Geometry: final body of the model. Coordinates: model frame, mm. Face numbers are marked on the shaded views. A direction names the side the tool comes from. Give positions to 0.01 mm unless a question says otherwise; leave off trailing zeros. Order: outer loops, then holes, each group sorted by start corner. A loop starts at its lowest first (then second) coordinate and runs counter-clockwise, first axis right, second up. Notation, with made-up numbers: (7.5, -31) -> (45.5, -31) arc R17 cw to (45.5, -26) -> close; hole circle Ø4 at (13.25, -23.75). An arc over 180 degrees is marked (long way). One line per question, with ' | ' between items.
from build123d import *

# Parameters (mm, degrees)
SKETCH1_W           = 60
SKETCH1_H           = 25
BOSS_EXTRUDE1_DEPTH = 6
CUT_EXTRUDE3_DEPTH  = 3
SKETCH5_R           = 1.15
CUT_EXTRUDE4_DEPTH  = 33.638167841
SKETCH7_W           = 60
SKETCH7_H           = 60
BOSS_EXTRUDE2_DEPTH = 4
SKETCH8_R           = 1.15
CUT_EXTRUDE5_DEPTH  = 10
CUT_EXTRUDE6_START  = -2
SKETCH9_R           = 1.15
CUT_EXTRUDE6_DEPTH  = 2


with BuildPart() as part:
    # Sketch1 → Boss-Extrude1 (new body)
    with BuildSketch(Plane.XY):
        Rectangle(SKETCH1_W, SKETCH1_H)
    extrude(amount=BOSS_EXTRUDE1_DEPTH)

    # Sketch4 → Cut-Extrude3 (cut)
    with BuildSketch(Plane(origin=(0, 0, 0), x_dir=(-1, 0, 0), z_dir=(0, 0, -1))):
        with BuildLine():
            ThreePointArc((8.45, 6), (4.86507576, 7.48492424), (6.35, 3.9))
            Line((6.35, 3.9), (6.35, 6))
            Line((6.35, 6), (8.45, 6))
        make_face()
        with BuildLine():
            Line((6.35, 6), (6.35, 3.9))
            ThreePointArc((6.35, 3.9), (7.83492424, 4.51507576), (8.45, 6))
            Line((8.45, 6), (6.35, 6))
        make_face()
        with BuildLine():
            ThreePointArc((12.25, 6), (12.86507576, 4.51507576), (14.35, 3.9))
            Line((14.35, 3.9), (14.35, 6))
            Line((14.35, 6), (12.25, 6))
        make_face()
        with BuildLine():
            Line((14.35, 6), (14.35, 3.9))
            ThreePointArc((14.35, 3.9), (15.83492424, 4.51507576), (16.45, 6))
            ThreePointArc((16.45, 6), (14.35, 8.1), (12.25, 6))
            Line((12.25, 6), (14.35, 6))
        make_face()
        with BuildLine():
            ThreePointArc((14.35, -3.9), (12.86507576, -4.51507576), (12.25, -6))
            Line((12.25, -6), (14.35, -6))
            Line((14.35, -6), (14.35, -3.9))
        make_face()
        with BuildLine():
            Line((14.35, -6), (12.25, -6))
            ThreePointArc((12.25, -6), (14.35, -8.1), (16.45, -6))
            ThreePointArc((16.45, -6), (15.83492424, -4.51507576), (14.35, -3.9))
            Line((14.35, -3.9), (14.35, -6))
        make_face()
        with BuildLine():
            Line((6.35, -3.9), (6.35, -6))
            Line((6.35, -6), (8.45, -6))
            ThreePointArc((8.45, -6), (7.83492424, -4.51507576), (6.35, -3.9))
        make_face()
        with BuildLine():
            Line((8.45, -6), (6.35, -6))
            Line((6.35, -6), (6.35, -3.9))
            ThreePointArc((6.35, -3.9), (4.86507576, -7.48492424), (8.45, -6))
        make_face()
    extrude(amount=-CUT_EXTRUDE3_DEPTH, mode=Mode.SUBTRACT)

    # Sketch5 → Cut-Extrude4 (cut, through all)
    with BuildSketch(Plane(origin=(0, 0, 3), x_dir=(-1, 0, 0), z_dir=(0, 0, -1))):
        with Locations((6.35, 6)):
            Circle(SKETCH5_R)
        with Locations((14.35, 6)):
            Circle(SKETCH5_R)
        with Locations((14.35, -6)):
            Circle(SKETCH5_R)
        with Locations((6.35, -6)):
            Circle(SKETCH5_R)
    extrude(amount=-CUT_EXTRUDE4_DEPTH, mode=Mode.SUBTRACT)

    # Sketch7 → Boss-Extrude2 (add)
    with BuildSketch(Plane(origin=(30, 0, 0), x_dir=(0, 0, -1), z_dir=(1, 0, 0))):
        with Locations((-3, 0)):
            Rectangle(SKETCH7_W, SKETCH7_H)
    extrude(amount=BOSS_EXTRUDE2_DEPTH)

    # Sketch8 → Cut-Extrude5 (cut)
    with BuildSketch(Plane(origin=(34, 0, 0), x_dir=(0, 0, -1), z_dir=(1, 0, 0))):
        with Locations(Location((-28, -25, 0), (0, 0, 90))):
            Circle(SKETCH8_R)
        with Locations(Location((-28, 25, 0), (0, 0, 90))):
            Circle(SKETCH8_R)
        with BuildLine():
            ThreePointArc((23.15, -25), (22.440085947, -23.937538538), (21.186827202, -24.186827202))
            Line((21.186827202, -24.186827202), (22.813172798, -25.813172798))
            ThreePointArc((22.813172798, -25.813172798), (23.062461462, -25.440085947), (23.15, -25))
        make_face()
        with BuildLine():
            Line((22.813172798, -25.813172798), (21.186827202, -24.186827202))
            ThreePointArc((21.186827202, -24.186827202), (21.186827202, -25.813172798), (22.813172798, -25.813172798))
        make_face()
        with Locations(Location((22, 25, 0), (0, 0, 90))):
            Circle(SKETCH8_R)
    extrude(amount=-CUT_EXTRUDE5_DEPTH, mode=Mode.SUBTRACT)

    # Sketch9 → Cut-Extrude6 (cut)
    # profile 1 of 6: a face of its own
    with BuildSketch(Plane.ZY.offset(-30).offset(CUT_EXTRUDE6_START)):
        Polygon((25.9, 26.212435565), (25.9, 23.787564435), (28, 22.575128869), (30.1, 23.787564435), (30.1, 26.212435565), (28, 27.424871131), align=None)
        with Locations(Location((28, 25, 0), (0, 0, 90))):
            Circle(SKETCH9_R, mode=Mode.SUBTRACT)
    # profile 2 of 6: a face of its own
    with BuildSketch(Plane.ZY.offset(-30).offset(CUT_EXTRUDE6_START)):
        with BuildLine():
            Line((28.813172798, -25.813172798), (29.537306696, -26.537306696))
            Line((29.537306696, -26.537306696), (30.1, -26.212435565))
            Line((30.1, -26.212435565), (30.1, -23.787564435))
            Line((30.1, -23.787564435), (28, -22.575128869))
            Line((28, -22.575128869), (26.462693304, -23.462693304))
            Line((26.462693304, -23.462693304), (27.186827202, -24.186827202))
            ThreePointArc((27.186827202, -24.186827202), (28.440085947, -23.937538538), (29.15, -25))
            ThreePointArc((29.15, -25), (29.062461462, -25.440085947), (28.813172798, -25.813172798))
        make_face()
    # profile 3 of 6: a face of its own
    with BuildSketch(Plane.ZY.offset(-30).offset(CUT_EXTRUDE6_START)):
        with BuildLine():
            Line((28, -27.424871131), (29.537306696, -26.537306696))
            Line((29.537306696, -26.537306696), (28.813172798, -25.813172798))
            ThreePointArc((28.813172798, -25.813172798), (27.186827202, -25.813172798), (27.186827202, -24.186827202))
            Line((27.186827202, -24.186827202), (26.462693304, -23.462693304))
            Line((26.462693304, -23.462693304), (25.9, -23.787564435))
            Line((25.9, -23.787564435), (25.9, -26.212435565))
            Line((25.9, -26.212435565), (28, -27.424871131))
        make_face()
    # profile 4 of 6: a face of its own
    with BuildSketch(Plane.ZY.offset(-30).offset(CUT_EXTRUDE6_START)):
        Polygon((-22, -22.575128869), (-24.1, -23.787564435), (-24.1, -26.212435565), (-22, -27.424871131), (-19.9, -26.212435565), (-19.9, -23.787564435), align=None)
        with Locations(Location((-22, -25, 0), (0, 0, 90))):
            Circle(SKETCH9_R, mode=Mode.SUBTRACT)
    # profile 5 of 6: a face of its own
    with BuildSketch(Plane.ZY.offset(-30).offset(CUT_EXTRUDE6_START)):
        with BuildLine():
            Line((-21.186827202, 24.186827202), (-20.462693304, 23.462693304))
            Line((-20.462693304, 23.462693304), (-19.9, 23.787564435))
            Line((-19.9, 23.787564435), (-19.9, 26.212435565))
            Line((-19.9, 26.212435565), (-22, 27.424871131))
            Line((-22, 27.424871131), (-23.537306696, 26.537306696))
            Line((-23.537306696, 26.537306696), (-22.813172798, 25.813172798))
            ThreePointArc((-22.813172798, 25.813172798), (-21.559914053, 26.062461462), (-20.85, 25))
            ThreePointArc((-20.85, 25), (-20.937538538, 24.559914053), (-21.186827202, 24.186827202))
        make_face()
    # profile 6 of 6: a face of its own
    with BuildSketch(Plane.ZY.offset(-30).offset(CUT_EXTRUDE6_START)):
        with BuildLine():
            Line((-22, 22.575128869), (-20.462693304, 23.462693304))
            Line((-20.462693304, 23.462693304), (-21.186827202, 24.186827202))
            ThreePointArc((-21.186827202, 24.186827202), (-22.813172798, 24.186827202), (-22.813172798, 25.813172798))
            Line((-22.813172798, 25.813172798), (-23.537306696, 26.537306696))
            Line((-23.537306696, 26.537306696), (-24.1, 26.212435565))
            Line((-24.1, 26.212435565), (-24.1, 23.787564435))
            Line((-24.1, 23.787564435), (-22, 22.575128869))
        make_face()
    extrude(amount=CUT_EXTRUDE6_DEPTH, mode=Mode.SUBTRACT)


solid = part.part
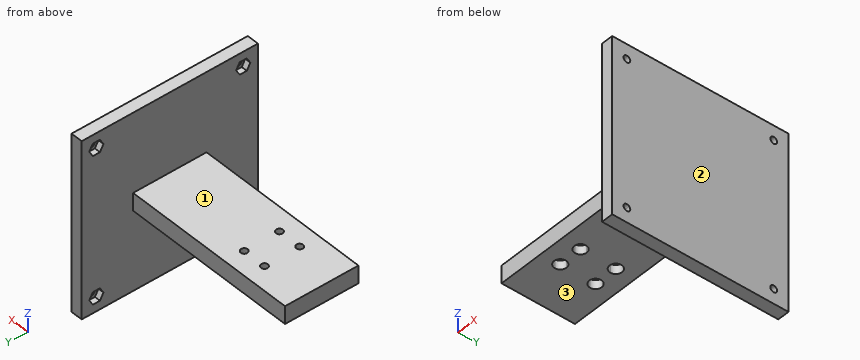
1) Contact query for flat-ended pins moving along their axis: pin 1 Ø5 at (x, y) = (-6, -5) entering from -Z; pin 2 Ø12.5 at (x, y) = (6.5, -1) entering from +Z; pin 3 Ø3.5 at (y, z) = (26, -23) entering from -X; pin 4 Ø1 at (x, y) = (8, -14) entering from -Z. Output: stop coordinate, or through.
Check result:
pin 1: stops at z = 0 | pin 2: stops at z = 6 | pin 3: stops at x = 30 | pin 4: passes through
2) Material intervals for probe 1 along Y at (x, z) = (33, 28); probe 2 along Y at (x, z) = (-6, 5); probe 3 along X at (y, z) = (26, 7), sorted ascending. Write a range as from..to.
Check result:
probe 1: y = -30..-26.15, -23.85..23.85, 26.15..30 | probe 2: y = -12.5..-7.1, -4.9..4.9, 7.1..12.5 | probe 3: x = 30..34
3) Section A-A on z = -16.5. Return loops of the section in (x, y).
Check result:
outline: (30, -30) -> (34, -30) -> (34, 30) -> (30, 30) -> close
4) Set-up query: the marked faces 1, 2 and 3. Return all of +Z, -Z, +X, -X, +Y, -Y with unobstructed straight access to the full face (end or side cutting, diameter ignored); none if empty.
Check result:
face 1: +Z, -X, +Y, -Y | face 2: +Z, -Z, +X, +Y, -Y | face 3: -Z, -X, +Y, -Y
5) Section B-B on y = -14. Return loops of the section in (x, z), plus the area to 3 significant figures.
Check result:
outline: (30, -27) -> (34, -27) -> (34, 33) -> (30, 33) -> close | area: 240 mm^2
